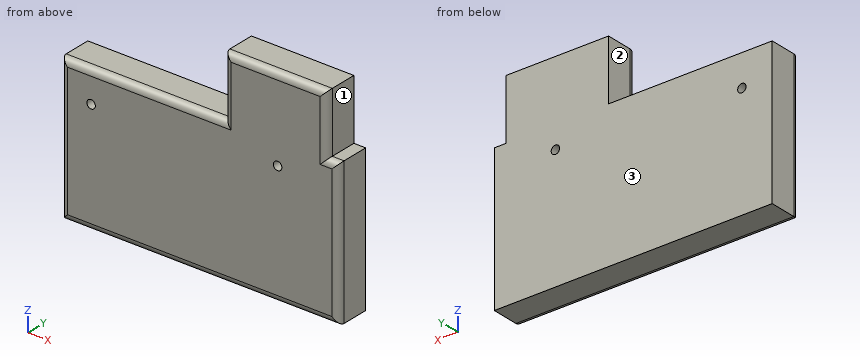
from build123d import *

# Parameters (mm, degrees)
F0_W     = 19.7901576757
F0_H     = 22.3555974662
F1_DEPTH = 25.4
F0_W_2   = 77.2351417691
F0_H_2   = 37.3888155445
F0_W_3   = 14.1860321164
F0_H_3   = 13.0779221654
F2_R     = 5.08
F4_R     = 14.5126216771
F5_DEPTH = 4.064
F7_D     = 6.35


with BuildPart() as f1:
    # F0 (on Front) → F1 (new body)
    with BuildSketch(Plane.XZ):
        Polygon((-143.1801915169, 45.9882542491), (-120.1951056719, 45.9882542491), (-120.1951056719, 68.3438517153), (-120.1951056719, 90.6994491816), (-143.1801915169, 90.6994491816), align=None)
        with Locations((-110.300026834, 79.5216504484)):
            Rectangle(F0_W, F0_H)
    extrude(amount=F1_DEPTH)


with BuildPart() as f1b:
    # F0 (on Front) → F1, piece 2 (new body)
    with BuildSketch(Plane.XZ):
        Polygon((23.0662133545, 45.1301448047), (-100.4049479961, 45.1301448047), (-100.4049479961, -64.0596598387), (109.2333272099, -64.0596598387), (109.2333272099, 45.1301448047), (100.3013551235, 45.1301448047), (100.3013551235, 7.7413292602), (23.0662133545, 7.7413292602), align=None)
        Polygon((23.0662133545, 90.6994491816), (23.0662133545, 45.1301448047), (100.3013551235, 45.1301448047), (100.3013551235, 90.6994491816), (88.216945529, 90.6994491816), (88.216945529, 77.6215270162), (74.0309134126, 77.6215270162), (74.0309134126, 90.6994491816), align=None)
        with Locations((61.683784239, 26.4357370324)):
            Rectangle(F0_W_2, F0_H_2)
        with Locations((81.1239294708, 84.1604880989)):
            Rectangle(F0_W_3, F0_H_3)
    extrude(amount=F1_DEPTH)

    # F2
    f2_edges = [f1b.edges().sort_by_distance(p)[0] for p in [
        (-38.669367, -25.4, 45.130145),
        (-100.404948, -25.4, -9.464758),
        (4.41419, -25.4, -64.05966),
        (109.233327, -25.4, -9.464758),
        (104.767341, -25.4, 45.130145),
        (100.301355, -25.4, 67.914797),
        (61.683784, -25.4, 90.699449),
        (23.066213, -25.4, 67.914797),
    ]]
    fillet(f2_edges, radius=F2_R)

    # F4 (on Front) → F5 (join)
    with BuildSketch(Plane.XZ):
        with Locations((-73.5853686929, -5.0210841)):
            Circle(F4_R)
    extrude(amount=F5_DEPTH)

    # F7 (through all)
    with Locations(Plane.XZ.offset(25.4)):
        with Locations((-77.5153413415, 21.2736316025), (63.1522908807, 28.0912686139)):
            Hole(F7_D / 2)


solid = f1b.part
Part model, mm, in its own coordinate system. Face numbers are marked on the shaded views. A direction names the side the tool comes from. Coordinates: 2 decimals unless noted, no trailing zeros. Loops run counter-clockwise (first coordinate to the right, second up) from the corner with the lowest first, then second, coordinate; pieces in that order, holes last. Notation, with made-up numbers: (33, 78.25) -> (75, 78.25) arc R26 cw to (75, 108.25) -> close; hole circle Ø1 at (54, -33). An arc over 180 degrees is marked (long way). Use a Markdown table: item, result. Add a question column.
Item 1: Which spindle directions (+Z, -Z, +X, -X, +Y, -Y) get a long thin tool onto all of the face, cutting with end or side? Do the marked faces 1, 2 and 3. Say none if no direction does.
Item 2: Band-saw the part on A-A on x = -78. Write the cut outline in (y, z).
Item 3: Flat gauge pins, fed straight in: P1, Ø10, axis at y = -6.5, z = 72, coming from the +X side; P2, Ø4.5, axis at x = 103, y = -13, coming from the +Z side; P3, Ø4, axis at y = -4.5, z = 53, coming from the -X side. Where does each tip first touch, or does it go through?
Item 4: Probe probe 1 along Z at (x, y) = (-46, -21); probe 2 along Z at (x, y) = (-63.5, -17.25); probe 3 along Z at (x, y) = (-75.5, -17.25). List the from-to ranges inside material, lowest first.
Item 5: Band-saw the part on B-B on y = -3.5. Write the cut outline in (x, z) (3 decimals), plus the area to 3 significant figures.
Item 6: Band-saw the part on C-C on z = 70. Write the cut outline in (x, y), plus the area to 3 significant figures.
Geometry says:
| question | item | result |
|---|---|---|
| 1 | face 1 | +Z, +X, +Y, -Y |
| 1 | face 2 | +Z, -X, +Y, -Y |
| 1 | face 3 | +Z, -Z, +X, -X, +Y |
| 2 | outline | (-25.4, -58.98) arc R5.08 ccw to (-20.32, -64.06) -> (0, -64.06) -> (0, 18.14) -> (-25.4, 18.14) -> close; (-25.4, 24.41) -> (0, 24.41) -> (0, 45.13) -> (-20.32, 45.13) arc R5.08 ccw to (-25.4, 40.05) -> close |
| 3 | P1 | x = 100.3 |
| 3 | P2 | z = 45.13 |
| 3 | P3 | x = 23.07 |
| 4 | probe 1 | -64.01 to 45.08 |
| 4 | probe 2 | -64.06 to 45.13 |
| 4 | probe 3 | -64.06 to 18.82, 23.73 to 45.13 |
| 5 | outline | (-100.405, -64.06) -> (109.233, -64.06) -> (109.233, 45.13) -> (100.301, 45.13) -> (100.301, 90.699) -> (23.066, 90.699) -> (23.066, 45.13) -> (-100.405, 45.13) -> close; hole circle Ø6.35 at (-77.515, 21.274); hole circle Ø6.35 at (63.152, 28.091) |
| 5 | area | 26,300 mm² |
| 6 | outline | (23.07, -20.32) arc R5.08 ccw to (28.15, -25.4) -> (95.22, -25.4) arc R5.08 ccw to (100.3, -20.32) -> (100.3, 0) -> (23.07, 0) -> close |
| 6 | area | 1,950 mm² |
